Geometry check sheet. Reference: the model listing, model coordinates, mm. Face numbers are marked on the shaded views. Round coordinates to 2 decimals unless told otherwise and drop trailing zeros. Write each loop counter-clockwise with the first axis right and the second up, starting at its lowest first coordinate (ties: lowest second). Pieces come first, ordered by that corner, then holes.
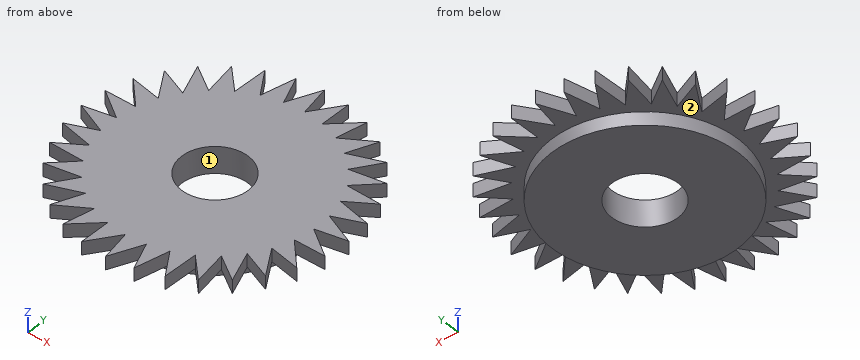
from build123d import *

# Parameters (mm, degrees)
Y_KSEKLIK_EKSTR_ZYON1_DEPTH = 1
IZIM3_R                     = 7
Y_KSEKLIK_EKSTR_ZYON2_DEPTH = 1
IZIM4_R                     = 2.5
KES_EKSTR_ZYON1_DEPTH       = 4


with BuildPart() as part:
    # Çizim1 → Yükseklik-Ekstrüzyon1 (new body)
    with BuildSketch(Plane.XY):
        Polygon((0, 10), (0.405515134, 7.700209394), (1.95090322, 9.807852804), (1.899959604, 7.473139952), (3.826834324, 9.238795325), (3.321389693, 6.958881932), (5.55570233, 8.314696123), (4.615180638, 6.177197982), (7.071067812, 7.071067812), (5.73161278, 5.158127778), (8.314696123, 5.55570233), (6.627782257, 3.940833616), (9.238795325, 3.826834324), (7.269249778, 2.572095429), (9.807852804, 1.95090322), (7.631364108, 1.104513056), (10, 0), (7.700209394, -0.405515134), (9.807852804, -1.95090322), (7.473139952, -1.899959604), (9.238795325, -3.826834324), (6.958881932, -3.321389693), (8.314696123, -5.55570233), (6.177197982, -4.615180638), (7.071067812, -7.071067812), (5.158127778, -5.73161278), (5.55570233, -8.314696123), (3.940833616, -6.627782257), (3.826834324, -9.238795325), (2.572095429, -7.269249778), (1.95090322, -9.807852804), (1.104513056, -7.631364108), (0, -10), (-0.405515134, -7.700209394), (-1.95090322, -9.807852804), (-1.899959604, -7.473139952), (-3.826834324, -9.238795325), (-3.321389693, -6.958881932), (-5.55570233, -8.314696123), (-4.615180638, -6.177197982), (-7.071067812, -7.071067812), (-5.73161278, -5.158127778), (-8.314696123, -5.55570233), (-6.627782257, -3.940833616), (-9.238795325, -3.826834324), (-7.269249778, -2.572095429), (-9.807852804, -1.95090322), (-7.631364108, -1.104513056), (-10, 0), (-7.700209394, 0.405515134), (-9.807852804, 1.95090322), (-7.473139952, 1.899959604), (-9.238795325, 3.826834324), (-6.958881932, 3.321389693), (-8.314696123, 5.55570233), (-6.177197982, 4.615180638), (-7.071067812, 7.071067812), (-5.158127778, 5.73161278), (-5.55570233, 8.314696123), (-3.940833616, 6.627782257), (-3.826834324, 9.238795325), (-2.572095429, 7.269249778), (-1.95090322, 9.807852804), (-1.104513056, 7.631364108), align=None)
    extrude(amount=Y_KSEKLIK_EKSTR_ZYON1_DEPTH)

    # Çizim3 → Yükseklik-Ekstrüzyon2 (add)
    with BuildSketch(Plane(origin=(0, 0, 0), x_dir=(-1, 0, 0), z_dir=(0, 0, -1))):
        Circle(IZIM3_R)
    extrude(amount=Y_KSEKLIK_EKSTR_ZYON2_DEPTH)

    # Çizim4 → Kes-Ekstrüzyon1 (cut)
    with BuildSketch(Plane(origin=(0, 0, -1), x_dir=(-1, 0, 0), z_dir=(0, 0, -1))):
        Circle(IZIM4_R)
    extrude(amount=-KES_EKSTR_ZYON1_DEPTH, mode=Mode.SUBTRACT)


solid = part.part
1. Section check A-A (z = -0.25). Record the cut outline in (x, y).
2. Scan lines: line 1 along Y through (x, z) = (0, -0.5); line 2 along X through (y, z) = (-9, 0.25); line 3 along X through (y, z) = (9, 0.95). Record each from-to range of solid material in increasing order.
3. Release check for a two-part mould opening along X. For the marked faces 1 and 2 record: +X half, -X half, draft (parallel to the pull), parting line (faces both ways), or undercut.
4. Depth check by flat-ended pin: pin 1 Ø4 at (x, y) = (7, 1.5) entering from -Z. Enter the tip coordinate at first touch or a pass-through.
Results below:
1. outline: circle Ø14 at (0, 0); hole circle Ø5 at (0, 0)
2. line 1: y = -7 to -2.5, 2.5 to 7
2. line 2: x = -3.77 to -3.57, -1.93 to -1.36, -0.18 to 0.47, 1.64 to 2.15, 3.67 to 3.84
2. line 3: x = -3.84 to -3.67, -2.15 to -1.64, -0.47 to 0.18, 1.36 to 1.93, 3.57 to 3.77
3. face 1: undercut
3. face 2: draft
4. pin 1: stops at z = -1
